Source: three-view drawing plus pictorial views. Frame: mm from the lowest corner of the part. Round coordinates to 2 decimals unless told otherwise and drop trailing zeros. Loops run counter-clockwise (first coordinate to the right, second up) from the corner with the lowest first, then second, coordinate; pieces in that order, holes last. Notation, with made-up numbers: (-34, 5.25) -> (-17, 5.25) arc R13 ccw to (-17, 20.25) -> close; hole circle Ø1 at (56.25, -39.5). An arc over 180 degrees is marked (long way). Answer as a JSON object with one key per item and string values. Group by question number.
Item 1: Section query D-D on x = 14.6. Return loops of the section in (y, z).
Item 2: Section query B-B on z = 5. Return loops of the section in (x, y), and give its area (3 significant figures).
Item 3: Material intervals for line 1 (Z direction, x = 9.8, y = 0.7); line 2 (Z direction, x = 14.6, y = 0.7); line 3 (X direction, y = 0.45, z = 4.5), sorted ascending. Write a range as [from, to].
Item 4: Draft query along Z for the marked faces 1, 2, 3 and 4. Return one class per face: released by +Z, released by -Z, zero draft, split by the parting line, or undercut.
Item 5: Section query A-A on x = 9.8. Return loops of the section in (y, z), and give its area (3 significant figures).
Item 6: Section query C-C on y = 1.7. Return loops of the section in (x, z).
Item 7: Pin query (flat end, axial travel): pin 1 (1.5 mm diameter, centred on x = 10, z = 4, fed in from -Y); pin 2 (1 mm diameter, centred on y = 1, z = 7.5, fed in from +X). Return the tip coordinate at first contact, or that it passes through.
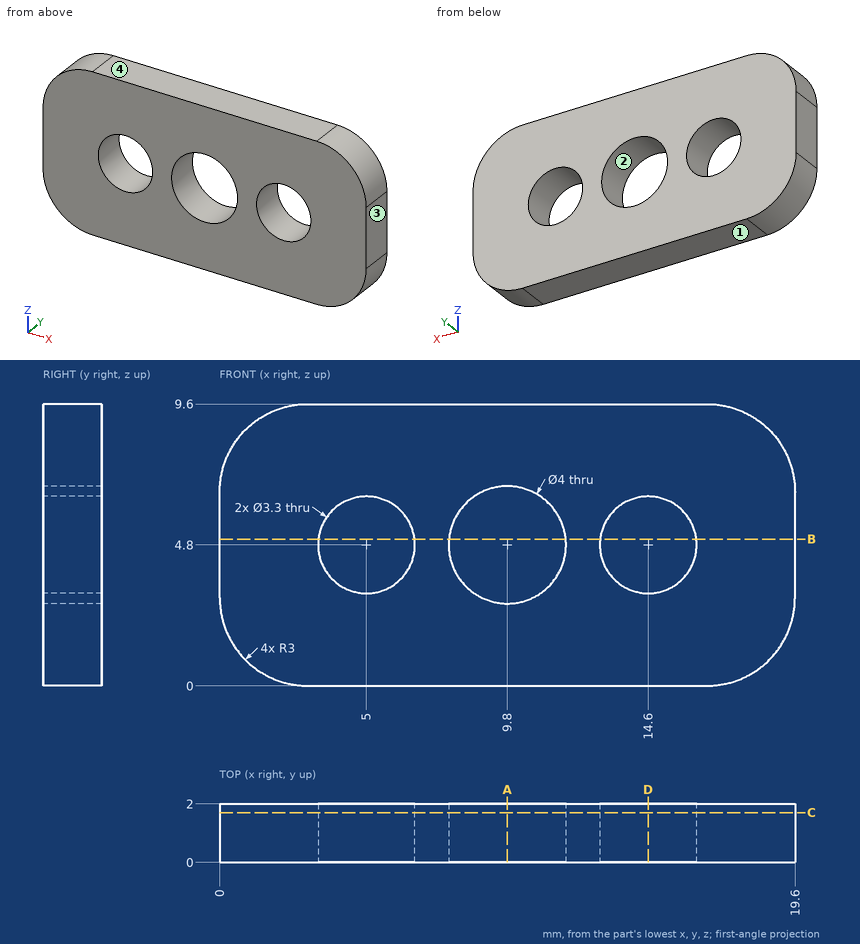
Solved:
{
 "1": {"outline": "(0, 0) -> (2, 0) -> (2, 3.15) -> (0, 3.15) -> close; (0, 6.45) -> (2, 6.45) -> (2, 9.6) -> (0, 9.6) -> close"},
 "2": {"outline": "(0, 0) -> (3.36, 0) -> (3.36, 2) -> (0, 2) -> close; (6.64, 0) -> (7.81, 0) -> (7.81, 2) -> (6.64, 2) -> close; (11.79, 0) -> (12.96, 0) -> (12.96, 2) -> (11.79, 2) -> close; (16.24, 0) -> (19.6, 0) -> (19.6, 2) -> (16.24, 2) -> close", "area": "18.1 mm²"},
 "3": {"line 1": "[0, 2.8], [6.8, 9.6]", "line 2": "[0, 3.15], [6.45, 9.6]", "line 3": "[0, 3.38], [6.62, 7.82], [11.78, 12.98], [16.22, 19.6]"},
 "4": {"face 1": "released by -Z", "face 2": "undercut", "face 3": "zero draft", "face 4": "released by +Z"},
 "5": {"outline": "(0, 0) -> (2, 0) -> (2, 2.8) -> (0, 2.8) -> close; (0, 6.8) -> (2, 6.8) -> (2, 9.6) -> (0, 9.6) -> close", "area": "11.2 mm²"},
 "6": {"outline": "(0, 3) arc R3 ccw to (3, 0) -> (16.6, 0) arc R3 ccw to (19.6, 3) -> (19.6, 6.6) arc R3 ccw to (16.6, 9.6) -> (3, 9.6) arc R3 ccw to (0, 6.6) -> close; hole circle Ø3.3 at (5, 4.8); hole circle Ø4 at (9.8, 4.8); hole circle Ø3.3 at (14.6, 4.8)"},
 "7": {"pin 1": "through", "pin 2": "x = 19.57"}
}
